For this review, take the finished solid that the model builds, in its own axes (mm). A direction names the side the tool comes from. Coordinates: 2 decimals unless noted, no trailing zeros. Loops run counter-clockwise (first coordinate to the right, second up) from the corner with the lowest first, then second, coordinate; pieces in that order, holes last. Notation, with made-up numbers: (-7, 28) - (40, 28) arc R15 cw to (40, 47) - close; hole circle Ø7 at (-34.5, 10.5). An arc over 180 degrees is marked (long way). One line per item, written item: value. Start each with the question number.
1. Take a section at A-A, the plane y = 4. State the section outline as (x, z) points.
2. Take a section at C-C, the plane y = 6. State the section outline as (x, z) points, and give its area (3 significant figures).
3. For faces 4 (the face through (10, 4, -1.5)), 5 (the face through (-5.22, 11.06, -2.67)), 6 (the face through (-5.229, 11.057, 2.657)), 7 (the face through (5.794, 11.057, -0.911)), list the 3-axis set-ups (+Z, -Z, +X, -X, +Y, -Y) from which the entire face can be reached by the end or side of a thin tool; tool diameter is ignored.
4. The part is to be moulded in two halves that separate along Z. For faces 1 (the face through (5.196, 11.057, 1.694)), 2 (the face through (0, 15.6, 2)), 3 (the face through (0.924, 11.057, -5.792)), say which applies: released by +Z, released by -Z, zero draft, split by the parting line, or undercut.
5. To check wall thickness, follow line 1 (X direction, y = 4.5, z = 0); line 2 (X direction, y = 6, z = 0); line 3 (Z direction, x = -1, y = 4.75). State the ranges of each line that lie inside material, in increasing order. Write a range as from..to.
6. Take a section at B-B, the plane x = 0. State the section outline as (y, z) points (3 decimals).
7. Insertion check: pin 1 (4 mm diameter, centred on x = 6, y = 12.5, fed in from -Z); pin 2 (8 mm diameter, centred on y = 7.5, z = 6, fed in from +X); pin 3 (1.8 mm diameter, centred on x = 0, z = 0, fed in from -Y); pin 4 (4 mm diameter, centred on x = 8, y = 3, fed in from -Z). Each pin has a flat end and moves straight along its axis. Give the tip position at first contact, or say it passes through.
```python
from build123d import *

# Parameters (mm, degrees)
SKETCH1_R           = 8
BOSS_EXTRUDE1_DEPTH = 8
SKETCH2_R           = 5.865
BOSS_EXTRUDE2_DEPTH = 6.2
CUT_EXTRUDE2_START  = -6.2
CUT_EXTRUDE2_DEPTH  = 6.2
SKETCH3_R           = 7.36
BOSS_EXTRUDE3_DEPTH = 1.4
CHAMFER1_SIZE       = 1.3
SKETCH4_R           = 2.75
BOSS_EXTRUDE4_DEPTH = 11
CUT_EXTRUDE1_DEPTH  = 2
SKETCH7_R           = 1.5
CUT_EXTRUDE3_DEPTH  = 21.696859757


with BuildPart() as part:
    # Sketch1 → Boss-Extrude1 (new body)
    with BuildSketch(Plane(origin=(0, 0, 0), x_dir=(1, 0, 0), z_dir=(0, 1, 0))):
        with Locations(Location((0, 0, 0), (0, 0, 270))):
            Circle(SKETCH1_R)
    extrude(amount=BOSS_EXTRUDE1_DEPTH)

    # Sketch2 → Boss-Extrude2 (add)
    with BuildSketch(Plane(origin=(0, 8, 0), x_dir=(1, 0, 0), z_dir=(0, 1, 0))):
        with Locations(Location((0, 0, 0), (0, 0, 90))):
            Circle(SKETCH2_R)
    extrude(amount=BOSS_EXTRUDE2_DEPTH)

    # Sketch6 → Cut-Extrude2 (cut)
    with BuildSketch(Plane(origin=(0, 14.2, 0), x_dir=(1, 0, 0), z_dir=(0, 1, 0)).offset(CUT_EXTRUDE2_START)):
        with BuildLine():
            Line((-0.460162596, 5.846920162), (-0.428778958, 5.448153229))
            ThreePointArc((-0.428778958, 5.448153229), (0, 5.465), (0.428778958, 5.448153229))
            Line((0.428778958, 5.448153229), (0.460162596, 5.846920162))
            ThreePointArc((0.460162596, 5.846920162), (0, 5.865), (-0.460162596, 5.846920162))
        make_face()
        with BuildLine():
            Line((2.244438331, 5.418553458), (2.091364958, 5.049001645))
            ThreePointArc((2.091364958, 5.049001645), (1.688777874, 5.197523862), (1.275778913, 5.314001615))
            Line((1.275778913, 5.314001615), (1.369157059, 5.702949583))
            ThreePointArc((1.369157059, 5.702949583), (1.812384672, 5.577946468), (2.244438331, 5.418553458))
        make_face()
        with BuildLine():
            Line((3.809012803, 4.459780988), (3.549233584, 4.155618602))
            ThreePointArc((3.549233584, 4.155618602), (3.212246404, 4.421277874), (2.855454656, 4.659678498))
            Line((2.855454656, 4.659678498), (3.064454082, 5.000734564))
            ThreePointArc((3.064454082, 5.000734564), (3.447360505, 4.744884672), (3.809012803, 4.459780988))
        make_face()
        with BuildLine():
            Line((5.000734564, 3.064454082), (4.659678498, 2.855454656))
            ThreePointArc((4.659678498, 2.855454656), (4.421277874, 3.212246404), (4.155618602, 3.549233584))
            Line((4.155618602, 3.549233584), (4.459780988, 3.809012803))
            ThreePointArc((4.459780988, 3.809012803), (4.744884672, 3.447360505), (5.000734564, 3.064454082))
        make_face()
        with BuildLine():
            Line((5.702949583, 1.369157059), (5.314001615, 1.275778913))
            ThreePointArc((5.314001615, 1.275778913), (5.197523862, 1.688777874), (5.049001645, 2.091364958))
            Line((5.049001645, 2.091364958), (5.418553458, 2.244438331))
            ThreePointArc((5.418553458, 2.244438331), (5.577946468, 1.812384672), (5.702949583, 1.369157059))
        make_face()
        with BuildLine():
            Line((5.846920162, -0.460162596), (5.448153229, -0.428778958))
            ThreePointArc((5.448153229, -0.428778958), (5.465, 0), (5.448153229, 0.428778958))
            Line((5.448153229, 0.428778958), (5.846920162, 0.460162596))
            ThreePointArc((5.846920162, 0.460162596), (5.865, 0), (5.846920162, -0.460162596))
        make_face()
        with BuildLine():
            Line((5.418553458, -2.244438331), (5.049001645, -2.091364958))
            ThreePointArc((5.049001645, -2.091364958), (5.197523862, -1.688777874), (5.314001615, -1.275778913))
            Line((5.314001615, -1.275778913), (5.702949583, -1.369157059))
            ThreePointArc((5.702949583, -1.369157059), (5.577946468, -1.812384672), (5.418553458, -2.244438331))
        make_face()
        with BuildLine():
            Line((4.459780988, -3.809012803), (4.155618602, -3.549233584))
            ThreePointArc((4.155618602, -3.549233584), (4.421277874, -3.212246404), (4.659678498, -2.855454656))
            Line((4.659678498, -2.855454656), (5.000734564, -3.064454082))
            ThreePointArc((5.000734564, -3.064454082), (4.744884672, -3.447360505), (4.459780988, -3.809012803))
        make_face()
        with BuildLine():
            Line((3.064454082, -5.000734564), (2.855454656, -4.659678498))
            ThreePointArc((2.855454656, -4.659678498), (3.212246404, -4.421277874), (3.549233584, -4.155618602))
            Line((3.549233584, -4.155618602), (3.809012803, -4.459780988))
            ThreePointArc((3.809012803, -4.459780988), (3.447360505, -4.744884672), (3.064454082, -5.000734564))
        make_face()
        with BuildLine():
            Line((1.369157059, -5.702949583), (1.275778913, -5.314001615))
            ThreePointArc((1.275778913, -5.314001615), (1.688777874, -5.197523862), (2.091364958, -5.049001645))
            Line((2.091364958, -5.049001645), (2.244438331, -5.418553458))
            ThreePointArc((2.244438331, -5.418553458), (1.812384672, -5.577946468), (1.369157059, -5.702949583))
        make_face()
        with BuildLine():
            Line((-0.460162596, -5.846920162), (-0.428778958, -5.448153229))
            ThreePointArc((-0.428778958, -5.448153229), (0, -5.465), (0.428778958, -5.448153229))
            Line((0.428778958, -5.448153229), (0.460162596, -5.846920162))
            ThreePointArc((0.460162596, -5.846920162), (0, -5.865), (-0.460162596, -5.846920162))
        make_face()
        with BuildLine():
            Line((-2.244438331, -5.418553458), (-2.091364958, -5.049001645))
            ThreePointArc((-2.091364958, -5.049001645), (-1.688777874, -5.197523862), (-1.275778913, -5.314001615))
            Line((-1.275778913, -5.314001615), (-1.369157059, -5.702949583))
            ThreePointArc((-1.369157059, -5.702949583), (-1.812384672, -5.577946468), (-2.244438331, -5.418553458))
        make_face()
        with BuildLine():
            Line((-3.809012803, -4.459780988), (-3.549233584, -4.155618602))
            ThreePointArc((-3.549233584, -4.155618602), (-3.212246404, -4.421277874), (-2.855454656, -4.659678498))
            Line((-2.855454656, -4.659678498), (-3.064454082, -5.000734564))
            ThreePointArc((-3.064454082, -5.000734564), (-3.447360505, -4.744884672), (-3.809012803, -4.459780988))
        make_face()
        with BuildLine():
            Line((-5.000734564, -3.064454082), (-4.659678498, -2.855454656))
            ThreePointArc((-4.659678498, -2.855454656), (-4.421277874, -3.212246404), (-4.155618602, -3.549233584))
            Line((-4.155618602, -3.549233584), (-4.459780988, -3.809012803))
            ThreePointArc((-4.459780988, -3.809012803), (-4.744884672, -3.447360505), (-5.000734564, -3.064454082))
        make_face()
        with BuildLine():
            Line((-5.702949583, -1.369157059), (-5.314001615, -1.275778913))
            ThreePointArc((-5.314001615, -1.275778913), (-5.197523862, -1.688777874), (-5.049001645, -2.091364958))
            Line((-5.049001645, -2.091364958), (-5.418553458, -2.244438331))
            ThreePointArc((-5.418553458, -2.244438331), (-5.577946468, -1.812384672), (-5.702949583, -1.369157059))
        make_face()
        with BuildLine():
            Line((-5.846920162, 0.460162596), (-5.448153229, 0.428778958))
            ThreePointArc((-5.448153229, 0.428778958), (-5.465, 0), (-5.448153229, -0.428778958))
            Line((-5.448153229, -0.428778958), (-5.846920162, -0.460162596))
            ThreePointArc((-5.846920162, -0.460162596), (-5.865, 0), (-5.846920162, 0.460162596))
        make_face()
        with BuildLine():
            Line((-5.418553458, 2.244438331), (-5.049001645, 2.091364958))
            ThreePointArc((-5.049001645, 2.091364958), (-5.197523862, 1.688777874), (-5.314001615, 1.275778913))
            Line((-5.314001615, 1.275778913), (-5.702949583, 1.369157059))
            ThreePointArc((-5.702949583, 1.369157059), (-5.577946468, 1.812384672), (-5.418553458, 2.244438331))
        make_face()
        with BuildLine():
            Line((-4.459780988, 3.809012803), (-4.155618602, 3.549233584))
            ThreePointArc((-4.155618602, 3.549233584), (-4.421277874, 3.212246404), (-4.659678498, 2.855454656))
            Line((-4.659678498, 2.855454656), (-5.000734564, 3.064454082))
            ThreePointArc((-5.000734564, 3.064454082), (-4.744884672, 3.447360505), (-4.459780988, 3.809012803))
        make_face()
        with BuildLine():
            Line((-3.064454082, 5.000734564), (-2.855454656, 4.659678498))
            ThreePointArc((-2.855454656, 4.659678498), (-3.212246404, 4.421277874), (-3.549233584, 4.155618602))
            Line((-3.549233584, 4.155618602), (-3.809012803, 4.459780988))
            ThreePointArc((-3.809012803, 4.459780988), (-3.447360505, 4.744884672), (-3.064454082, 5.000734564))
        make_face()
        with BuildLine():
            Line((-1.369157059, 5.702949583), (-1.275778913, 5.314001615))
            ThreePointArc((-1.275778913, 5.314001615), (-1.688777874, 5.197523862), (-2.091364958, 5.049001645))
            Line((-2.091364958, 5.049001645), (-2.244438331, 5.418553458))
            ThreePointArc((-2.244438331, 5.418553458), (-1.812384672, 5.577946468), (-1.369157059, 5.702949583))
        make_face()
    extrude(amount=CUT_EXTRUDE2_DEPTH, mode=Mode.SUBTRACT)

    # Sketch3 → Boss-Extrude3 (add)
    with BuildSketch(Plane(origin=(0, 14.2, 0), x_dir=(1, 0, 0), z_dir=(0, 1, 0))):
        with Locations(Location((0, 0, 0), (0, 0, 270))):
            Circle(SKETCH3_R)
    extrude(amount=BOSS_EXTRUDE3_DEPTH)

    # Chamfer1
    chamfer1_edges = [part.edges().sort_by_distance(p)[0] for p in [
        (0, 14.2, -7.36),
    ]]
    chamfer(chamfer1_edges, length=CHAMFER1_SIZE)

    # Sketch4 → Boss-Extrude4 (add)
    with BuildSketch(Plane(origin=(0, 0, 0), x_dir=(0, 0, -1), z_dir=(1, 0, 0))):
        with Locations(Location((0, 4, 0), (0, 0, 180))):
            Circle(SKETCH4_R)
    extrude(amount=BOSS_EXTRUDE4_DEPTH)

    # Sketch5 → Cut-Extrude1 (cut)
    with BuildSketch(Plane(origin=(11, 0, 0), x_dir=(0, 0, -1), z_dir=(1, 0, 0))):
        Polygon((0, 2.267949192), (1.5, 3.133974596), (1.5, 4.866025404), (0, 5.732050808), (-1.5, 4.866025404), (-1.5, 3.133974596), align=None)
    extrude(amount=-CUT_EXTRUDE1_DEPTH, mode=Mode.SUBTRACT)

    # Sketch7 → Cut-Extrude3 (cut, through all)
    with BuildSketch(Plane.XZ):
        with Locations(Location((0, 0, 0), (0, 0, 270))):
            Circle(SKETCH7_R)
    extrude(amount=-CUT_EXTRUDE3_DEPTH, mode=Mode.SUBTRACT)


solid = part.part
```
Solutions:
1. outline: (7.51, -2.75) - (11, -2.75) - (11, -1.5) - (9, -1.5) - (9, 1.5) - (11, 1.5) - (11, 2.75) - (7.51, 2.75) arc R8 ccw (long way) to start; hole circle Ø3 at (0, 0)
2. outline: (7.77, -1.89) - (11, -1.89) - (11, 1.89) - (7.77, 1.89) arc R8 ccw (long way) to start; hole circle Ø3 at (0, 0)
2. area: 206 mm2
3. face 4: +X
3. face 5: -Z, -X
3. face 6: +Z, -X
3. face 7: -Z, +X
4. face 1: undercut
4. face 2: zero draft
4. face 3: released by -Z
5. line 1: -8..-1.5, 1.5..9
5. line 2: -8..-1.5, 1.5..11
5. line 3: -7.94..-1.12, 1.12..7.94
6. outline: (0, -8) - (8, -8) - (8, -5.465) - (14.2, -5.465) - (14.2, -6.06) - (15.5, -7.36) - (15.6, -7.36) - (15.6, -1.5) - (0, -1.5) - close; (0, 1.5) - (15.6, 1.5) - (15.6, 7.36) - (15.5, 7.36) - (14.2, 6.06) - (14.2, 5.465) - (8, 5.465) - (8, 8) - (0, 8) - close
7. pin 1: z = -4.29
7. pin 2: x = 7.75
7. pin 3: through
7. pin 4: z = -5.29
